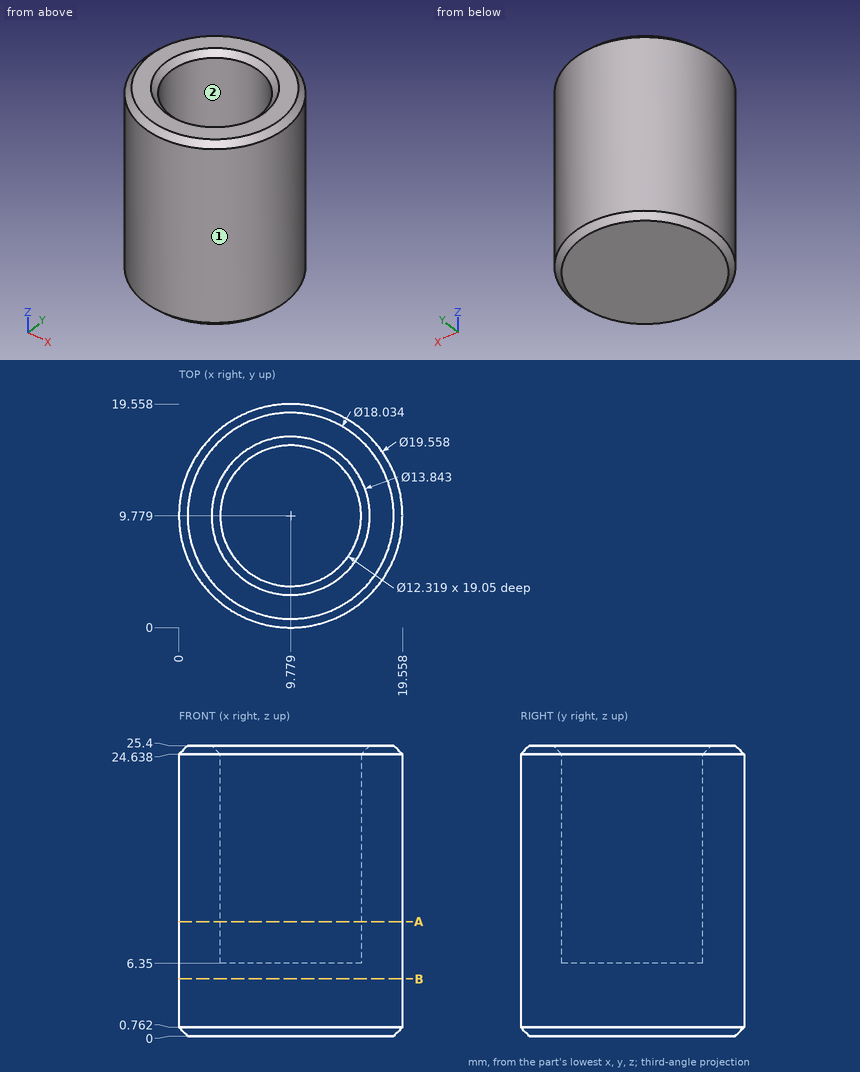
Geometry check sheet. Reference: drawing and pictorial views, mm from the part's lowest x, y, z. A direction names the side the tool comes from. Round coordinates to 2 decimals unless told otherwise and drop trailing zeros. Write each loop counter-clockwise with the first axis right and the second up, starting at its lowest first coordinate (ties: lowest second). Pieces come first, ordered by that corner, then holes.
(1) Section check A-A (z = 10). Enter the section's corners in (x, y).
Returned:
outline: circle Ø19.56 at (9.78, 9.78); hole circle Ø12.32 at (9.78, 9.78)
(2) Section check B-B (z = 5). Enter the section's corners in (x, y), plus the area to 3 significant figures.
Returned:
outline: circle Ø19.56 at (9.78, 9.78)
area: 300 mm2
(3) Material ranges on line 1 (Y direction, x = 9.5, z = 14.25); line 2 (Z direction, x = 7.25, y = 7.5), recorded low to high.
Returned:
line 1: y = 0 to 3.63, 15.93 to 19.55
line 2: z = 0 to 6.35
(4) Access from +Z, -Z, +X, -X, +Y, -Y to the whole of each face (thin tool, end or side, straight path). Record for the marked faces 1 and 2.
Returned:
face 1: +Z, -Z
face 2: +Z
(5) Depth check by flat-ended pin: pin 1 Ø11 at (x, y) = (9.779, 9.779) entering from +Z; pin 2 Ø1 at (x, z) = (4.5, 4) entering from -Y; pin 3 Ø1.5 at (x, z) = (7.5, 6) entering from +Y. Enter the tip coordinate at first touch or a pass-through.
Returned:
pin 1: stops at z = 6.35
pin 2: stops at y = 1.25
pin 3: stops at y = 19.44
